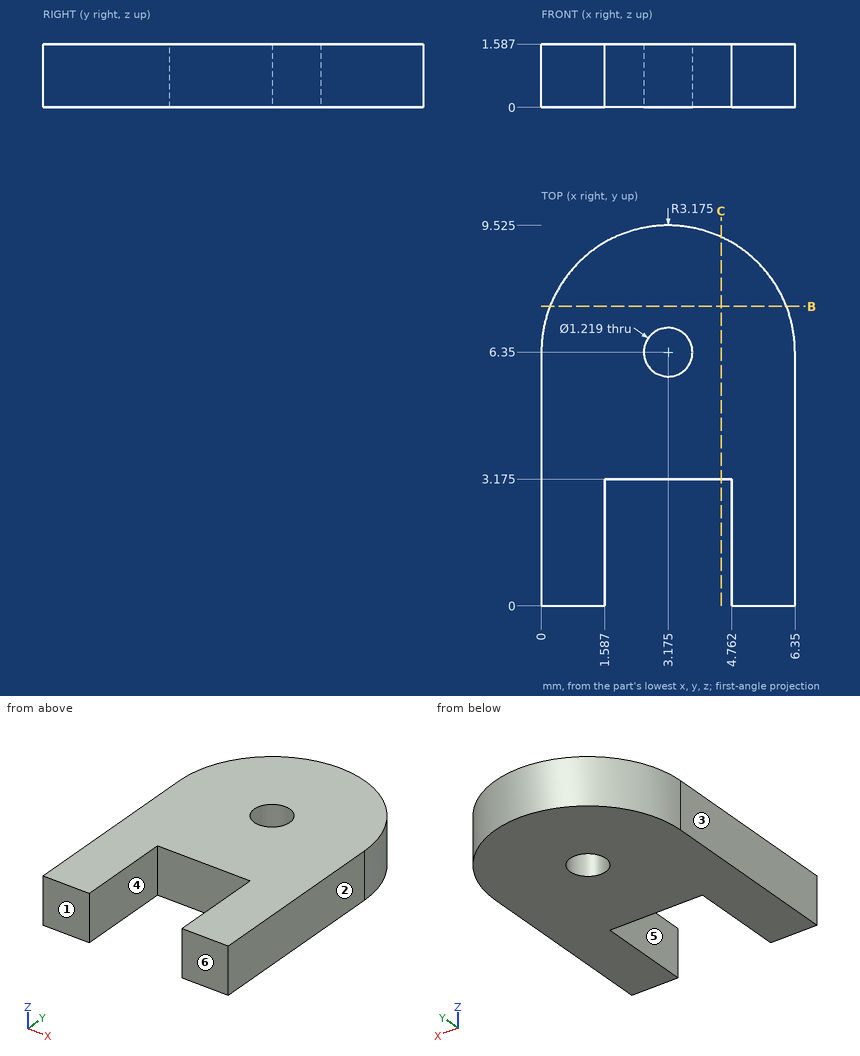
For this review, use the dimensioned drawing (mm, ordinates from the lowest corner) and the shaded views. A direction names the side the tool comes from. Round coordinates to 2 decimals unless told otherwise and drop trailing zeros. Loops run counter-clockwise (first coordinate to the right, second up) from the corner with the lowest first, then second, coordinate; pieces in that order, holes last. Notation, with made-up numbers: (20.5, 25.25) -> (75.5, 25.25) arc R33 ccw to (75.5, 56.25) -> close; hole circle Ø4 at (-31, -14.75). An arc over 180 degrees is marked (long way). Write item = value, one per line. Start each with the question number.
Item 1: To check wall thickness, follow L1, parallel to X at y = 1.5, z = 1; L2, parallel to Y at x = 2.75, z = 1.05 (1 decimal); L3, parallel to X at y = 6.5, z = 1.55 (1 decimal). State the ranges of each line that lie inside material, in increasing order.
Item 2: Mouldability with a two-part tool opening along X and no side actions: class the marked faces 1, 2, 3 and 4 as released by +X, released by -X, zero draft, split by the parting line, or undercut.
Item 3: Insertion check: pin 1 (0.8 mm diameter, centred on x = 4, z = 1, fed in from -Y) (1 decimal). The pin has a flat end and moves straight along its axis. Give the tip position at first contact, or say it passes through.
Item 4: Take a section at B-B on y = 7.5. Give the boundary of the cut face in (x, z) (1 decimal).
Item 5: Take a section at C-C on x = 4.5. Give the boundary of the cut face in (y, z) (1 decimal).
Item 6: For the marked faces 5 and 6, list the 3-axis set-ups (+Z, -Z, +X, -X, +Y, -Y) from which the entire face can be reached by the end or side of a thin tool; tool diameter is ignored.
Result:
q1.L1 = 0 to 1.59, 4.76 to 6.35
q1.L2 = 3.2 to 5.9, 6.8 to 9.5
q1.L3 = 0 to 2.6, 3.8 to 6.3
q2.face_1 = zero draft
q2.face_2 = released by +X
q2.face_3 = released by -X
q2.face_4 = undercut
q3.pin_1 = 3.2
q4.outline = (0.2, 0) -> (6.1, 0) -> (6.1, 1.6) -> (0.2, 1.6) -> close
q5.outline = (3.2, 0) -> (9.2, 0) -> (9.2, 1.6) -> (3.2, 1.6) -> close
q6.face_5 = +Z, -Z, -Y
q6.face_6 = +Z, -Z, +X, -X, -Y
